The listing builds one solid part. Answer for the finished solid, in the listing's coordinates (mm). Round coordinates to 2 decimals unless told otherwise and drop trailing zeros. Order: outer loops, then holes, each group sorted by start corner. A loop starts at its lowest first (then second) coordinate and runs counter-clockwise, first axis right, second up. Notation, with made-up numbers: (2, 36) - (61, 36) arc R28 cw to (61, 71) - close; hole circle Ø5 at (5, 67). An arc over 180 degrees is marked (long way). Use CSV: the item, a comma, the result in double quotes. Start each with the question number.
Item 1: Straight lines are drawn through the part: line 1 along X through (y, z) = (-125, 0.75); line 2 along Y through (x, z) = (2, 1.9); line 3 along X through (y, z) = (56, 2.4). For each, find the intervals that lie inside material, in ascending order. Write a range as [from, to].
Item 2: Find section C-C, the plane z = 1.75. Count the separate pieces of the cut face and the enclosed holes in it, plus the area to 3 significant figures.
Item 3: Find section B-B, the plane x = -18. Give the vertices of the cut face in (y, z).
Item 4: Find section A-A, the plane y = 55. Give the vertices of the cut face in (x, z).
Item 5: Find section D-D, the plane x = -50.5. Give the vertices of the cut face in (y, z), plus the area to 3 significant figures.
```python
from build123d import *

# Parameters (mm, degrees)
MAIN_DEPTH                      = 3
SKETCH2_R                       = 12
SKETCH2_R_2                     = 1.5
SKETCH2_R_3                     = 10
SINGLEHOLES_DEPTH               = 4
SKETCH3_R                       = 1.5
TOPLEFTHOLE_DEPTH               = 4
TOPLEFT2HOLELINEARPATTERN_COUNT = 6
TOPLEFT2HOLELINEARPATTERN_PITCH = 20
SKETCH4_R                       = 1.5
TOPLEFT1HOLE_DEPTH              = 4
TOPLEFT1HOLELINEARPATTERN_COUNT = 5
TOPLEFT1HOLELINEARPATTERN_PITCH = 20
SKETCH5_R                       = 1.5
TOPRIGHTHOLE_DEPTH              = 4
TOPRIGHTHOLELINEARPATTERN_COUNT = 5
TOPRIGHTHOLELINEARPATTERN_PITCH = 20
MOTORHOLEFIXSKETCH_R            = 1.5
MOTORHOLEFIX_DEPTH              = 4
MOTORHOLEFIXLINEARPATTERN_COUNT = 3
MOTORHOLEFIXLINEARPATTERN_PITCH = 20
SKETCH6_R                       = 1.5
CUT_EXTRUDE1_DEPTH              = 4


with BuildPart() as part:
    # Sketch1 → Main (new body)
    with BuildSketch(Plane.XY):
        Polygon((-60, 110), (-60, 0), (20, 0), (20, 20), (40, 40), (40, 130), (-40, 130), align=None)
        Polygon((-25, 100), (-15, 100), (-15, 127), (15, 127), (15, 100), (25, 100), (25, 70), (-25, 70), align=None, mode=Mode.SUBTRACT)
    extrude(amount=MAIN_DEPTH)

    # Sketch2 → SingleHoles (cut, through all)
    with BuildSketch(Plane.XY.offset(3)):
        with Locations((-35, 0)):
            Circle(SKETCH2_R)
        with Locations((-55, 0)):
            Circle(SKETCH2_R_2)
        with Locations((22.5, 55)):
            Circle(SKETCH2_R_3)
        Circle(SKETCH2_R_2)
        with Locations((-45, 115)):
            Circle(SKETCH2_R_2)
        with Locations((22.5, 35)):
            Circle(SKETCH2_R_2)
    extrude(amount=-SINGLEHOLES_DEPTH, mode=Mode.SUBTRACT)

    # Sketch3 → TopLeftHole (cut, through all)
    with BuildSketch(Plane.XY.offset(3)):
        with Locations((-35, 125)):
            Circle(SKETCH3_R)
    toplefthole = extrude(amount=-TOPLEFTHOLE_DEPTH, mode=Mode.SUBTRACT)

    # TopLeft2HoleLinearPattern: TopLeftHole ×6
    with Locations(*[(0, -i * TOPLEFT2HOLELINEARPATTERN_PITCH, 0) for i in range(1, TOPLEFT2HOLELINEARPATTERN_COUNT)]):
        add(toplefthole, mode=Mode.SUBTRACT)

    # Sketch4 → TopLeft1Hole (cut, through all)
    with BuildSketch(Plane.XY.offset(3)):
        with Locations((-35, 105)):
            Circle(SKETCH4_R)
        with Locations((-55, 105)):
            Circle(SKETCH4_R)
    topleft1hole = extrude(amount=-TOPLEFT1HOLE_DEPTH, mode=Mode.SUBTRACT)

    # TopLeft1HoleLinearPattern: TopLeft1Hole ×5
    with Locations(*[(0, -i * TOPLEFT1HOLELINEARPATTERN_PITCH, 0) for i in range(1, TOPLEFT1HOLELINEARPATTERN_COUNT)]):
        add(topleft1hole, mode=Mode.SUBTRACT)

    # Sketch5 → TopRightHole (cut, through all)
    with BuildSketch(Plane.XY.offset(3)):
        with Locations((35, 125)):
            Circle(SKETCH5_R)
    toprighthole = extrude(amount=-TOPRIGHTHOLE_DEPTH, mode=Mode.SUBTRACT)

    # TopRightHoleLinearPattern: TopRightHole ×5
    with Locations(*[(0, -i * TOPRIGHTHOLELINEARPATTERN_PITCH, 0) for i in range(1, TOPRIGHTHOLELINEARPATTERN_COUNT)]):
        add(toprighthole, mode=Mode.SUBTRACT)

    # MotorHoleFixSketch → MotorHoleFix (cut, through all)
    with BuildSketch(Plane.XY.offset(3)):
        with Locations((0, 65)):
            Circle(MOTORHOLEFIXSKETCH_R)
        with Locations((-10, 65)):
            Circle(MOTORHOLEFIXSKETCH_R)
        with Locations((10, 65)):
            Circle(MOTORHOLEFIXSKETCH_R)
    motorholefix = extrude(amount=-MOTORHOLEFIX_DEPTH, mode=Mode.SUBTRACT)

    # MotorHoleFixLinearPattern: MotorHoleFix ×3
    with Locations(*[(0, -i * MOTORHOLEFIXLINEARPATTERN_PITCH, 0) for i in range(1, MOTORHOLEFIXLINEARPATTERN_COUNT)]):
        add(motorholefix, mode=Mode.SUBTRACT)

    # Sketch6 → Cut-Extrude1 (cut, through all)
    with BuildSketch(Plane.XY.offset(3)):
        with Locations((25, 125)):
            Circle(SKETCH6_R)
        with Locations((25, 105)):
            Circle(SKETCH6_R)
    cut_extrude1 = extrude(amount=-CUT_EXTRUDE1_DEPTH, mode=Mode.SUBTRACT)

    # Mirror1: Cut-Extrude1 across plane
    add(cut_extrude1.mirror(Plane(origin=(0, 0, 0), x_dir=(0, 0, 1), z_dir=(1, 0, 0))), mode=Mode.SUBTRACT)

    # LeftRightMirror: part across plane


with BuildPart() as part_1:
    add(part.part)
    add(part.part.mirror(Plane.ZX))


solid = part_1.part
```
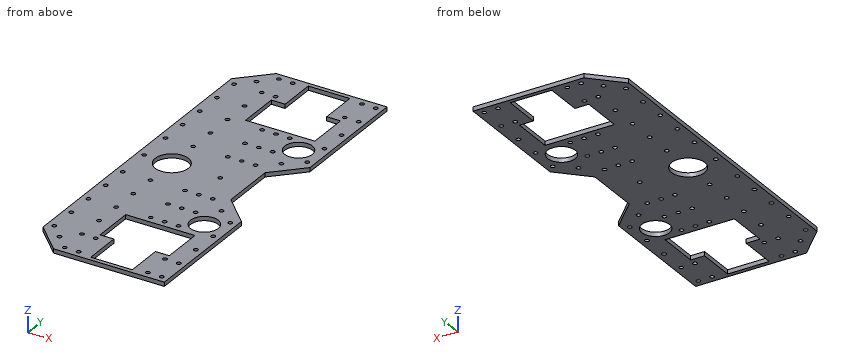
Worked out:
1,line 1,"x = [-45, -36.5], [-33.5, -26.5], [-23.5, -15], [15, 23.5], [26.5, 33.5], [36.5, 40]"
1,line 2,"y = [-130, -127], [-70, 70], [127, 130]"
1,line 3,"x = [-60, 12.55], [32.45, 40]"
2,separate pieces,"1"
2,enclosed holes,"69"
2,area,"18,200 mm²"
3,outline,"(-130, 0) - (-100, 0) - (-100, 3) - (-130, 3) - close; (-70, 0) - (70, 0) - (70, 3) - (-70, 3) - close; (100, 0) - (130, 0) - (130, 3) - (100, 3) - close"
4,outline,"(-60, 0) - (12.5, 0) - (12.5, 3) - (-60, 3) - close; (32.5, 0) - (40, 0) - (40, 3) - (32.5, 3) - close"
5,outline,"(-119.5, 0) - (119.5, 0) - (119.5, 3) - (-119.5, 3) - close"
5,area,"717 mm²"
